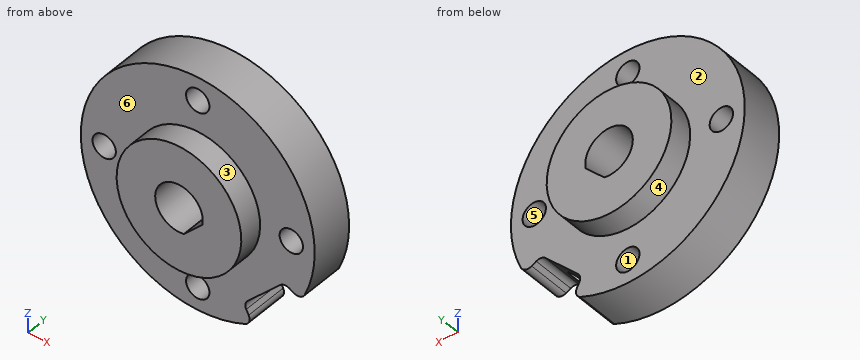
from build123d import *

# Parameters (mm, degrees)
SKETCH_1_R               = 15
SKETCH_1_R_2             = 2
SKETCH_1_R_3             = 1.5
EXTRUDE_1_DEPTH          = 3
EXTRUDE_2_DEPTH          = 4.25
EXTRUDE_2_DEPTH_BACK     = 7.25
SKETCH_2_R               = 8
EXTRUDE_3_DEPTH          = 1.25
EXTRUDE_3_DEPTH_BACK     = 4.25
SKETCH_5_R               = 15
CUT_EXTRUDE_1_DEPTH      = 5
CUT_EXTRUDE_1_DEPTH_BACK = 16.5
SKETCH_6_R               = 1.3
CUT_EXTRUDE_2_DEPTH      = 14
SKETCH_7_R               = 1.5
CUT_EXTRUDE_4_DEPTH      = 14
CUT_EXTRUDE_START        = -14
CUT_EXTRUDE_5_DEPTH      = 14
FILLET_1_R               = 1


with BuildPart() as part:
    # 草图1 → 凸台-拉伸1 (new body)
    with BuildSketch(Plane(origin=(0, 0, 0), x_dir=(1, 0, 0), z_dir=(0, 1, 0))):
        with Locations(Location((0, 0, 0), (0, 0, 270))):
            Circle(SKETCH_1_R)
        with Locations(Location((0, 0, 0), (0, 0, 270))):
            Circle(SKETCH_1_R_2, mode=Mode.SUBTRACT)
        with Locations(Location((0, 6, 0), (0, 0, 270))):
            Circle(SKETCH_1_R_3, mode=Mode.SUBTRACT)
        with Locations(Location((6, 0, 0), (0, 0, 270))):
            Circle(SKETCH_1_R_3, mode=Mode.SUBTRACT)
        with Locations(Location((0, -6, 0), (0, 0, 270))):
            Circle(SKETCH_1_R_3, mode=Mode.SUBTRACT)
        with Locations(Location((-6, 0, 0), (0, 0, 270))):
            Circle(SKETCH_1_R_3, mode=Mode.SUBTRACT)
        with Locations(Location((0, 12, 0), (0, 0, 270))):
            Circle(SKETCH_1_R_3, mode=Mode.SUBTRACT)
        with Locations(Location((12, 0, 0), (0, 0, 270))):
            Circle(SKETCH_1_R_3, mode=Mode.SUBTRACT)
        with Locations(Location((0, -12, 0), (0, 0, 270))):
            Circle(SKETCH_1_R_3, mode=Mode.SUBTRACT)
        with Locations(Location((-12, 0, 0), (0, 0, 270))):
            Circle(SKETCH_1_R_3, mode=Mode.SUBTRACT)
    extrude(amount=EXTRUDE_1_DEPTH)

    # 草图2 → 凸台-拉伸2 (add, two sides: drawn at the far end of the back side and taken through both)
    with BuildSketch(Plane.XZ.offset(-EXTRUDE_2_DEPTH_BACK)):
        with Locations(Location((0, 0, 0), (0, 0, 270))):
            Circle(SKETCH_2_R)
    extrude(amount=EXTRUDE_2_DEPTH + EXTRUDE_2_DEPTH_BACK)

    # 草图5 → 凸台-拉伸3 (add, two sides: drawn at the far end of the back side and taken through both)
    with BuildSketch(Plane(origin=(0, 3, 0), x_dir=(1, 0, 0), z_dir=(0, 1, 0)).offset(-EXTRUDE_3_DEPTH_BACK)):
        with Locations(Location((0, 0, 0), (0, 0, 270))):
            Circle(SKETCH_5_R)
    extrude(amount=EXTRUDE_3_DEPTH + EXTRUDE_3_DEPTH_BACK)

    # 草图3 → 切除-拉伸1 (cut, two sides: drawn at the far end of the back side and taken through both)
    with BuildSketch(Plane(origin=(0, 3, 0), x_dir=(1, 0, 0), z_dir=(0, 1, 0)).offset(-CUT_EXTRUDE_1_DEPTH_BACK)):
        with BuildLine():
            Line((0.619906335, 2.986338249), (2.986338249, 0.619906335))
            ThreePointArc((2.986338249, 0.619906335), (-2.156675683, -2.156675683), (0.619906335, 2.986338249))
        make_face()
    extrude(amount=CUT_EXTRUDE_1_DEPTH + CUT_EXTRUDE_1_DEPTH_BACK, mode=Mode.SUBTRACT)

    # 草图6 → 切除-拉伸2 (cut)
    with BuildSketch(Plane(origin=(1.803122292, 0, -1.803122292), x_dir=(0.7071067811865465, 0, 0.7071067811865486), z_dir=(-0.7071067811865486, 0, 0.7071067811865465))):
        with Locations((0, 1.5)):
            Circle(SKETCH_6_R)
    extrude(amount=-CUT_EXTRUDE_2_DEPTH, mode=Mode.SUBTRACT)

    # 草图7 → 切除-拉伸4 (cut)
    with BuildSketch(Plane(origin=(0, 7.25, 0), x_dir=(1, 0, 0), z_dir=(0, 1, 0))):
        with Locations(Location((0, 12, 0), (0, 0, 270))):
            Circle(SKETCH_7_R)
        with Locations(Location((-12, 0, 0), (0, 0, 270))):
            Circle(SKETCH_7_R)
        with Locations(Location((12, 0, 0), (0, 0, 270))):
            Circle(SKETCH_7_R)
        with Locations(Location((0, -12, 0), (0, 0, 270))):
            Circle(SKETCH_7_R)
    extrude(amount=-CUT_EXTRUDE_4_DEPTH, mode=Mode.SUBTRACT)

    # 草图8 → 切除-拉伸5 (cut)
    with BuildSketch(Plane(origin=(0, 4.25, 0), x_dir=(1, 0, 0), z_dir=(0, 1, 0)).offset(CUT_EXTRUDE_START)):
        with BuildLine():
            Line((7.02021556, 13.255812819), (5.875756654, 11.094806094))
            Line((5.875756654, 11.094806094), (11.094806094, 5.875756654))
            Line((11.094806094, 5.875756654), (13.255812819, 7.02021556))
            ThreePointArc((13.255812819, 7.02021556), (10.606601718, 10.606601718), (7.02021556, 13.255812819))
        make_face()
    extrude(amount=CUT_EXTRUDE_5_DEPTH, mode=Mode.SUBTRACT)

    # 圆角1
    fillet_1_edges = [part.edges().sort_by_distance(p)[0] for p in [
        (13.255812819, 1.5, -7.02021556),
        (5.875756654, 1.5, -11.094806094),
        (7.02021556, 1.5, -13.255812819),
        (11.094806094, 1.5, -5.875756654),
    ]]
    fillet(fillet_1_edges, radius=FILLET_1_R)


solid = part.part
The model under review builds one solid part; all positions refer to its coordinate system, in mm. Face numbers are marked on the shaded views. A direction names the side the tool comes from. Round coordinates to 2 decimals unless told otherwise and drop trailing zeros. Order: outer loops, then holes, each group sorted by start corner. A loop starts at its lowest first (then second) coordinate and runs counter-clockwise, first axis right, second up. Notation, with made-up numbers: (88.25, -3) -> (138.25, -3) arc R26 ccw to (138.25, 17) -> close; hole circle Ø8 at (2, 81.5). An arc over 180 degrees is marked (long way). Return JSON: item names as keys, results as strings.
1. For the marked faces 1, 2 and 3, list the 3-axis set-ups (+Z, -Z, +X, -X, +Y, -Y) from which the entire face can be reached by the end or side of a thin tool; tool diameter is ignored.
Answer block:
{"face 1": "+Y, -Y", "face 2": "+Y", "face 3": "-Y"}
2. For L1, parallel to X at y = 2.05, z = 0; L2, parallel to Y at x = 4.5, z = 7.5; L3, parallel to Z at x = -11, y = 0.5, list the stretches that pass through material, from the lowest coordinate up. Write a range as [from, to].
Answer block:
{"L1": "x = [-15, -13.5], [-10.5, -3.05], [3.05, 10.5], [13.5, 15]", "L2": "y = [-1.25, 4.25]", "L3": "z = [-10.2, -1.12], [1.12, 10.2]"}
3. Insertion check: P1, Ø2, axis at y = 3.5, z = -2.5, coming from the -X side; P2, Ø5, axis at x = -9, z = 9, coming from the +Y side; P3, Ø5, axis at y = 4, z = -2, coming from the -X side; P4, Ø3, axis at y = 2, z = -11, coming from the +X side. Each pin has a flat end and moves straight along its axis. Give the tip position at first contact, or say it passes through.
Answer block:
{"P1": "stops at x = -14.92", "P2": "stops at y = 4.25", "P3": "stops at x = -15", "P4": "stops at x = 7.47"}
4. Take a section at D-D (x = 0). Write out the cut boundary in (y, z), then the cut area to 3 significant figures.
Answer block:
{"outline": "(-4.25, -8) -> (-1.25, -8) -> (-1.25, -10.5) -> (4.25, -10.5) -> (4.25, -8) -> (7.25, -8) -> (7.25, -3.05) -> (-4.25, -3.05) -> close; (-4.25, 3.05) -> (7.25, 3.05) -> (7.25, 8) -> (4.25, 8) -> (4.25, 10.5) -> (-1.25, 10.5) -> (-1.25, 8) -> (-4.25, 8) -> close; (-1.25, -15) -> (4.25, -15) -> (4.25, -13.5) -> (-1.25, -13.5) -> close; (-1.25, 13.5) -> (4.25, 13.5) -> (4.25, 15) -> (-1.25, 15) -> close", "area": "158 mm²"}
5. Take a section at B-B (x = -12). Write out the cut boundary in (y, z).
Answer block:
{"outline": "(-1.25, -9) -> (4.25, -9) -> (4.25, -1.5) -> (-1.25, -1.5) -> close; (-1.25, 1.5) -> (4.25, 1.5) -> (4.25, 9) -> (-1.25, 9) -> close"}
6. The part is to be moulded in two halves that separate along X. For the marked faces 4, 5 and 6, say which applies: +X half, -X half, draft (parallel to the pull), parting line (faces both ways), or undercut.
Answer block:
{"face 4": "parting line", "face 5": "undercut", "face 6": "draft"}
7. Take a section at A-A (z = 12). Write out the cut boundary in (x, y).
Answer block:
{"outline": "(-9, -1.25) -> (-1.5, -1.25) -> (-1.5, 4.25) -> (-9, 4.25) -> close; (1.5, -1.25) -> (9, -1.25) -> (9, 4.25) -> (1.5, 4.25) -> close"}
8. Take a section at C-C (y = 3.25). Write out the cut boundary in (x, z).
Answer block:
{"outline": "(6.06, -13.72) arc R1 ccw to (6.54, -12.34) -> (6.22, -11.75) arc R1 cw to (6.4, -10.57) -> (10.57, -6.4) arc R1 cw to (11.75, -6.22) -> (12.34, -6.54) arc R1 ccw to (13.72, -6.06) arc R15 ccw (long way) to start; hole circle Ø3 at (-12, 0); hole circle Ø3 at (0, -12); hole circle Ø3 at (0, 12); hole (0.62, -2.99) -> (2.99, -0.62) arc R3.05 ccw (long way) to start; hole circle Ø3 at (12, 0)"}
